```python
from build123d import *

# Parameters (mm, degrees)
SKETCH1_W               = 298.45
SKETCH1_H               = 152.4
BOSS_EXTRUDE1_DEPTH     = 4.7625
CUT_EXTRUDE2_DEPTH      = 168.825106137
F_10_CLEARANCE_HOLE3_D  = 5.1054
LPATTERN2_COUNT         = 4
LPATTERN2_PITCH         = 63.5
F_10_32_TAPPED_HOLE1_D  = 4.0386
F_1_4_CLEARANCE_HOLE1_D = 6.7564


with BuildPart() as part:
    # Sketch1 → Boss-Extrude1 (new, symmetric)
    with BuildSketch(Plane(origin=(0, 0, 0), x_dir=(1, 0, 0), z_dir=(0, 1, 0))):
        Rectangle(SKETCH1_W, SKETCH1_H)
    extrude(amount=BOSS_EXTRUDE1_DEPTH, both=True)

    # Sketch4 → Cut-Extrude2 (cut, through all)
    with BuildSketch(Plane.XZ.offset(4.7625)):
        with BuildLine():
            Line((-107.315, 33.9979), (107.315, 33.9979))
            ThreePointArc((107.315, 33.9979), (109.5629, 31.75), (107.315, 29.5021))
            Line((107.315, 29.5021), (-107.315, 29.5021))
            ThreePointArc((-107.315, 29.5021), (-109.5629, 31.75), (-107.315, 33.9979))
        make_face()
        with BuildLine():
            Line((-107.315, 8.5979), (107.315, 8.5979))
            ThreePointArc((107.315, 8.5979), (109.5629, 6.35), (107.315, 4.1021))
            Line((107.315, 4.1021), (-107.315, 4.1021))
            ThreePointArc((-107.315, 4.1021), (-109.5629, 6.35), (-107.315, 8.5979))
        make_face()
    extrude(amount=-CUT_EXTRUDE2_DEPTH, mode=Mode.SUBTRACT)

    # #10 Clearance Hole3 (through all)
    with Locations(Plane(origin=(0, 4.7625, 0), x_dir=(1, 0, 0), z_dir=(0, 1, 0))):
        with Locations((-95.25, 60.325)):
            f_10_clearance_hole3 = Hole(F_10_CLEARANCE_HOLE3_D / 2)

    # LPattern2: #10 Clearance Hole3 ×4
    with Locations(*[(i * LPATTERN2_PITCH, 0, 0) for i in range(1, LPATTERN2_COUNT)]):
        add(f_10_clearance_hole3, mode=Mode.SUBTRACT)

    # #10-32 Tapped Hole1 (through all)
    with Locations(Plane(origin=(0, 4.7625, 0), x_dir=(1, 0, 0), z_dir=(0, 1, 0))):
        with Locations((-139.7, -14.605), (139.7, -14.605)):
            Hole(F_10_32_TAPPED_HOLE1_D / 2)

    # 1/4 Clearance Hole1 (through all)
    with Locations(Plane(origin=(0, 4.7625, 0), x_dir=(1, 0, 0), z_dir=(0, 1, 0))):
        with Locations((-65.0875, 19.05), (-26.9875, 19.05)):
            f_1_4_clearance_hole1 = Hole(F_1_4_CLEARANCE_HOLE1_D / 2)

    # Mirror5: 1/4 Clearance Hole1 across plane
    add(f_1_4_clearance_hole1.mirror(Plane(origin=(0, 0, 0), x_dir=(0, 0, 1), z_dir=(1, 0, 0))), mode=Mode.SUBTRACT)


solid = part.part
```
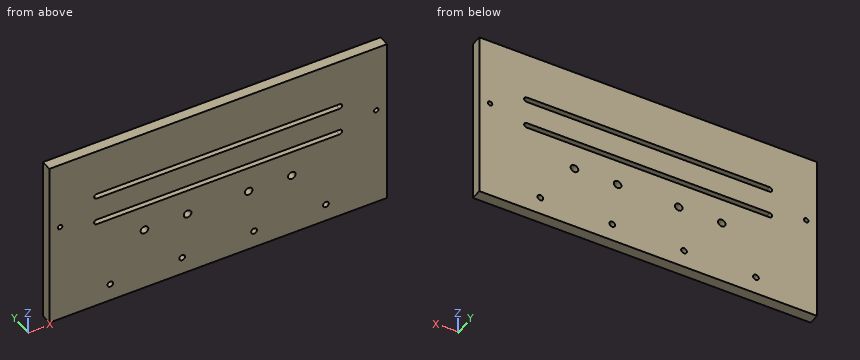
Check sheet for the modelled part. Datum: model origin and axes. Units: mm. Round coordinates to 2 decimals unless told otherwise and drop trailing zeros. Loops run counter-clockwise (first coordinate to the right, second up) from the corner with the lowest first, then second, coordinate; pieces in that order, holes last. Notation, with made-up numbers: (80, -6.75) - (137, -6.75) arc R19 cw to (137, 10.25) - close; hole circle Ø6 at (-27, -21). An arc over 180 degrees is marked (long way). Answer as a JSON object with one key per item and string values. Group by question number.
Q1. Scan lines: line 1 along Z through (x, y) = (59, -2.75); line 2 along Z through (x, y) = (-95.25, -0.5); line 3 along X through (y, z) = (2.75, -60) (3 decimals). Record each from-to range of solid material in increasing order. Write a range as [from, to].
Q2. Sectioned sample at C-C, the plane y = -1.25. Count the separate pieces of the cut face and the enclosed holes in it, plus the area to 3 significant figures.
Q3. Sectioned sample at A-A, the plane z = -19.05. Enter the section's corners in (x, y) (1 decimal).
Q4. Sectioned sample at B-B, the plane x = -73. Enter the section's corners in (y, z).
Q5. Gauge pin test, flat end, axial feed: P1, Ø2.5, axis at x = -139.7, z = 14.605, coming from the +Y side. Record the tip position at first contact, or that the pin passes through.
Solution:
{
 "1": {"line 1": "z = [-76.2, 4.1], [8.6, 29.5], [34, 76.2]", "line 2": "z = [-76.2, -62.88], [-57.77, 4.1], [8.6, 29.5], [34, 76.2]", "line 3": "x = [-149.225, -97.782], [-92.718, -34.282], [-29.218, 29.218], [34.282, 92.718], [97.782, 149.225]"},
 "2": {"separate pieces": "1", "enclosed holes": "12", "area": "43,300 mm²"},
 "3": {"outline": "(-149.2, -4.8) - (-68.5, -4.8) - (-68.5, 4.8) - (-149.2, 4.8) - close; (-61.7, -4.8) - (-30.4, -4.8) - (-30.4, 4.8) - (-61.7, 4.8) - close; (-23.6, -4.8) - (23.6, -4.8) - (23.6, 4.8) - (-23.6, 4.8) - close; (30.4, -4.8) - (61.7, -4.8) - (61.7, 4.8) - (30.4, 4.8) - close; (68.5, -4.8) - (149.2, -4.8) - (149.2, 4.8) - (68.5, 4.8) - close"},
 "4": {"outline": "(-4.76, -76.2) - (4.76, -76.2) - (4.76, 4.1) - (-4.76, 4.1) - close; (-4.76, 8.6) - (4.76, 8.6) - (4.76, 29.5) - (-4.76, 29.5) - close; (-4.76, 34) - (4.76, 34) - (4.76, 76.2) - (-4.76, 76.2) - close"},
 "5": {"P1": "passes through"}
}
